Here's how the part is built. I have some questions about the finished solid (model axes, mm). Face numbers are marked on the shaded views. Give positions to 0.01 mm unless a question says otherwise; leave off trailing zeros. Loops run counter-clockwise (first coordinate to the right, second up) from the corner with the lowest first, then second, coordinate; pieces in that order, holes last.
Q1. I need wall thicknesses on line 1 (Y direction, x = 27.5, z = 13.25); line 2 (X direction, y = -15, z = 17.25); line 3 (Z direction, x = 44, y = -21.3). Which ranges of each line are inside material? Lowest first, please.
Q2. If we section it at C-C (x = -44): Please give me the cut outline in (y, z), plus the area to 3 significant figures.
Q3. If we section it at A-A (x = 27.5): Please give me the cut outline in (y, z).
Q4. If we section it at B-B (y = 3.5): Please give me the cut outline in (x, z), plus the area to 3 significant figures.
Q5. We'd pull the mould along Y, two halves only. Please class the marked faces 1, 2 and 3: +Y half, -Y half, draft (parallel to the pull), parting line (faces both ways), or undercut.
Q6. Will this pin go through, and if not, where does the flat tip stop? P1, Ø3, axis at x = -44.5, z = 15.5, coming from the -Y side.
Q7. If we section it at D-D (z = 28.25): Please give me the cut outline in (x, y), plus the area to 3 significant figures.
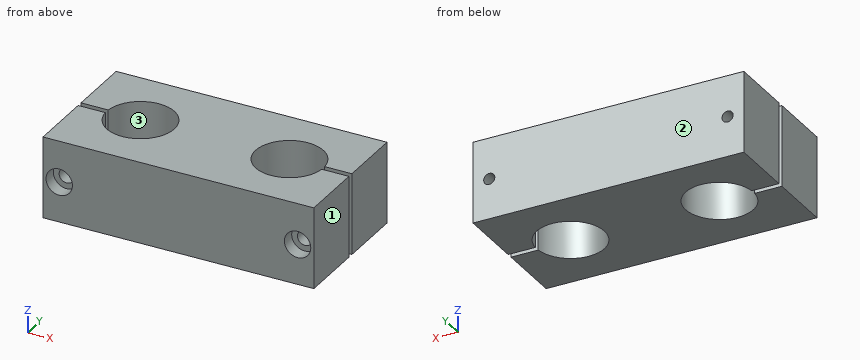
from build123d import *

# Parameters (mm, degrees)
F1_DEPTH       = 30
F3_D           = 5.5
F3_DEPTH       = 25
F3_CBORE_D     = 9.75
F3_CBORE_DEPTH = 5
F3_TIP         = 1.6523667023
F5_D           = 4.1


with BuildPart() as f1:
    # F0 (on Top) → F1 (new body)
    with BuildSketch(Plane.XY):
        with BuildLine():
            Line((50, 1), (50, 25))
            Line((50, 25), (-50, 25))
            Line((-50, 25), (-50, 1))
            Line((-50, 1), (-39.9599357944, 1))
            ThreePointArc((-39.9599357944, 1), (-15, 0), (-39.9599357944, -1))
            Line((-39.9599357944, -1), (-50, -1))
            Line((-50, -1), (-50, -25))
            Line((-50, -25), (50, -25))
            Line((50, -25), (50, -1))
            Line((50, -1), (39.9599357944, -1))
            ThreePointArc((39.9599357944, -1), (15, 0), (39.9599357944, 1))
            Line((39.9599357944, 1), (50, 1))
        make_face()
    extrude(amount=F1_DEPTH)

    # F3
    with Locations(Plane.XZ.offset(25)):
        with Locations((-44, 14.8143433034), (44, 14.8143433034)):
            CounterBoreHole(F3_D / 2, F3_CBORE_D / 2, F3_CBORE_DEPTH, depth=F3_DEPTH)
            with Locations((0, 0, -(F3_DEPTH + F3_TIP / 2))):  # 118° drill point
                Cone(0, F3_D / 2, F3_TIP, mode=Mode.SUBTRACT)

    # F5 (through all)
    with Locations(Plane.XZ.offset(-1)):
        with Locations((-44, 14.8143433034), (44, 14.8143433034)):
            Hole(F5_D / 2)


solid = f1.part
Check sheet entries:
1. line 1: y = -25 to -12.5, 12.5 to 25
1. line 2: x = -50 to -45.28, -42.72 to 42.72, 45.28 to 50
1. line 3: z = 0 to 9.94, 19.69 to 30
2. outline: (-25, 0) - (-1, 0) - (-1, 12.06) - (-20, 12.06) - (-20, 9.94) - (-25, 9.94) - close; (-25, 19.69) - (-20, 19.69) - (-20, 17.56) - (-1, 17.56) - (-1, 30) - (-25, 30) - close; (1, 0) - (25, 0) - (25, 12.76) - (1, 12.76) - close; (1, 16.86) - (25, 16.86) - (25, 30) - (1, 30) - close
2. area: 1,190 mm2
3. outline: (-25, 0) - (-12.5, 0) - (-12.5, 30) - (-25, 30) - close; (12.5, 0) - (25, 0) - (25, 30) - (12.5, 30) - close
4. outline: (-50, 0) - (-39.5, 0) - (-39.5, 30) - (-50, 30) - close; (-15.5, 0) - (15.5, 0) - (15.5, 30) - (-15.5, 30) - close; (39.5, 0) - (50, 0) - (50, 30) - (39.5, 30) - close; hole circle Ø4.1 at (-44, 14.81); hole circle Ø4.1 at (44, 14.81)
4. area: 1,530 mm2
5. face 1: draft
5. face 2: +Y half
5. face 3: undercut
6. P1: stops at y = 1
7. outline: (-50, -25) - (50, -25) - (50, -1) - (39.96, -1) arc R12.5 cw (long way) to (39.96, 1) - (50, 1) - (50, 25) - (-50, 25) - (-50, 1) - (-39.96, 1) arc R12.5 cw (long way) to (-39.96, -1) - (-50, -1) - close
7. area: 3,980 mm2
